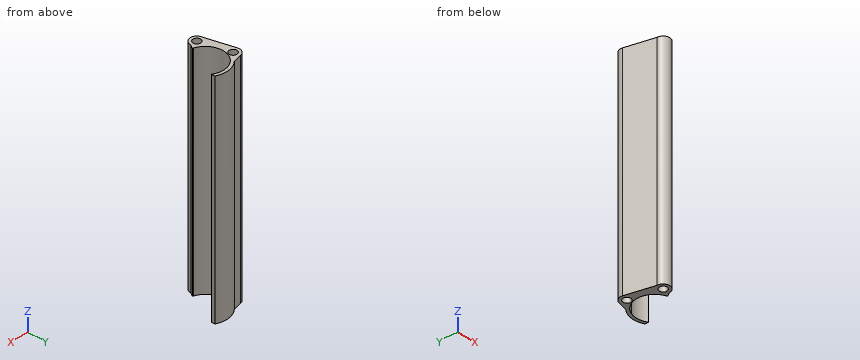
```python
from build123d import *

# Parameters (mm, degrees)
ESQUISSE1_R        = 2.625
BOSS_EXTRU_1_DEPTH = 150


with BuildPart() as part:
    # Esquisse1 → Boss.-Extru.1 (new body)
    with BuildSketch(Plane.XY):
        with BuildLine():
            ThreePointArc((-0.79755539, 4.428758901), (-3.787637609, 2.429773929), (-4.358021192, -1.12145053))
            Line((-4.358021192, -1.12145053), (0.5, -20))
            ThreePointArc((0.5, -20), (5, -24.5), (9.5, -20))
            Line((9.5, -20), (11.28572177, -17.287605871))
            ThreePointArc((11.28572177, -17.287605871), (10.940890985, -17.183131081), (10.599214607, -17.068761049))
            ThreePointArc((10.599214607, -17.068761049), (2.237966256, -5.391928791), (10.376689651, 6.441078731))
            ThreePointArc((10.376689651, 6.441078731), (16.104400227, 7.151408987), (21.540678755, 5.212823607))
            Line((21.540678755, 5.212823607), (21.540678755, 7.531281515))
            ThreePointArc((21.540678755, 7.531281515), (13.221135766, 9.146884287), (5.419576542, 5.836198326))
            Line((5.419576542, 5.836198326), (-0.79755539, 4.428758901))
        make_face()
        with Locations((5, -20)):
            Circle(ESQUISSE1_R, mode=Mode.SUBTRACT)
        Circle(ESQUISSE1_R, mode=Mode.SUBTRACT)
    extrude(amount=BOSS_EXTRU_1_DEPTH)


solid = part.part
```
Build history of the part. All positions in model axes, mm. Coordinates: 2 decimals unless noted, no trailing zeros. Order: outer loops, then holes, each group sorted by start corner. A loop starts at its lowest first (then second) coordinate and runs counter-clockwise, first axis right, second up.
Item 1: Saw through at B-B on y = -5. List the corners of the cut face in (x, z).
Filled in:
outline: (-3.36, 0) - (2.24, 0) - (2.24, 150) - (-3.36, 150) - close
Item 2: Drill centre lines: L1, parallel to Y at x = 6.75, z = 112; L2, parallel to Y at x = 5, z = 68 (3 decimals); L3, parallel to Y at x = 1.75, z = 28.5. Where is each one in solid material? Low to high.
Filled in:
L1: y = -24.15 to -21.96, -18.04 to -14.89, 4.34 to 6.83
L2: y = -24.5 to -22.625, -17.375 to -13.112, 2.564 to 5.741
L3: y = -23.11 to -1.96, 1.96 to 5.01
Item 3: Drop flat-ended pins along their axis: pin 1 Ø10 at (x, z) = (6.5, 61.5) entering from +Y; pin 2 Ø8 at (y, z) = (-6.5, 95.5) entering from +X; pin 3 Ø4.5 at (x, y) = (0, 0) entering from -Z; pin 4 Ø3 at (x, y) = (0.5, -20.5) entering from +Z. Give the stop position or say it passes through.
Filled in:
pin 1: stops at y = 8.86
pin 2: stops at x = 3.38
pin 3: passes through
pin 4: stops at z = 150
Item 4: Saw through at A-A on z = 20. List the corners of the cut face in (x, y) (3 decimals), then the cut area to 3 significant figures.
Filled in:
outline: (-4.358, -1.121) - (0.5, -20) arc R4.5 ccw to (9.5, -20) - (11.286, -17.288) arc R12.5 cw (long way) to (21.541, 5.213) - (21.541, 7.531) arc R14.5 ccw to (5.42, 5.836) - (-0.798, 4.429) arc R4.5 ccw to start; hole circle Ø5.25 at (0, 0); hole circle Ø5.25 at (5, -20)
area: 203 mm2
